Part print with two shaded views. Sizes in mm from the minimum x, y, z corner. A direction names the side the tool comes from. Round coordinates to 2 decimals unless told otherwise and drop trailing zeros. Loops run counter-clockwise (first coordinate to the right, second up) from the corner with the lowest first, then second, coordinate; pieces in that order, holes last. Notation, with made-up numbers: (8.5, 36) - (56.5, 36) arc R29 ccw to (56.5, 58) - close; hole circle Ø3 at (33, 23). An arc over 180 degrees is marked (long way). Write each question's results on one line, items separated by ' | '. Start each with the question number.
(1) Cut at C-C, the plane x = 74.5. List the corners of the cut face in (y, z).
(2) Cut at A-A, the plane z = 118. List the corners of the cut face in (x, y), then the cut area to 3 significant figures.
(3) Tool access for the marked faces 1 and 2: list every direction of +Z, -Z, +X, -X, +Y, -Y with a clear straight run to the whole face (end or side of a thin tool).
(4) Cut at B-B, the plane y = 435. List the corners of the cut face in (x, z), then the cut area to 3 significant figures.
(5) Drill centre lines: L1, parallel to X at y = 181, z = 215; L2, parallel to Y at x = 305, z = 185.5; L3, parallel to Z at x = 333.5, y = 365.5. Where is each one in solid material? Low to high.
(6) Mould opens along X. For the marked faces 3, 4, 5 and 6 say: released by +X, released by -X, zero draft, split by the parting line, or undercut.
(7) Flat gauge pin, fed straight in: P1, Ø6, axis at x = 337, y = 106, coming from the +Z side. Where does the tip first touch, or does it go through?
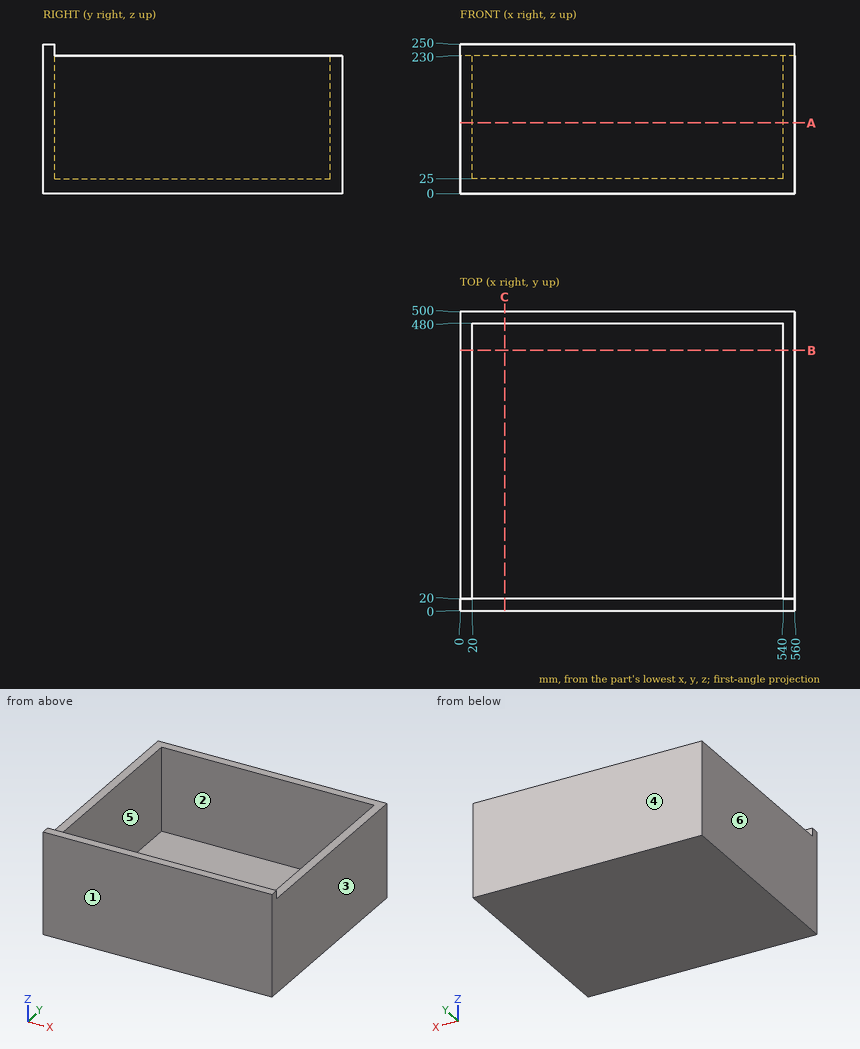
A:
1) outline: (0, 0) - (500, 0) - (500, 230) - (480, 230) - (480, 25) - (20, 25) - (20, 250) - (0, 250) - close
2) outline: (0, 0) - (560, 0) - (560, 500) - (0, 500) - close; hole (20, 20) - (540, 20) - (540, 480) - (20, 480) - close | area: 40,800 mm2
3) face 1: +Z, -Z, +X, -X, -Y | face 2: +Z
4) outline: (0, 0) - (560, 0) - (560, 230) - (540, 230) - (540, 25) - (20, 25) - (20, 230) - (0, 230) - close | area: 22,200 mm2
5) L1: 0 to 20, 540 to 560 | L2: 0 to 20, 480 to 500 | L3: 0 to 25
6) face 3: released by +X | face 4: zero draft | face 5: undercut | face 6: released by -X
7) P1: z = 25
